Source: CAD feature listing. Evaluate the final solid. Frame: model axes, mm. A direction names the side the tool comes from. Give positions to 0.01 mm unless a question says otherwise; leave off trailing zeros. Write each loop counter-clockwise with the first axis right and the second up, starting at its lowest first coordinate (ties: lowest second). Pieces come first, ordered by that corner, then holes.
```python
from build123d import *

# Parameters (mm, degrees)
SKETCH2_R           = 1.5875
BOSS_EXTRUDE1_DEPTH = 1.6
SKETCH3_W           = 15.875
SKETCH3_H           = 16.4592
BOSS_EXTRUDE2_DEPTH = 12.5


with BuildPart() as part:
    # Sketch2 → Boss-Extrude1 (new body)
    with BuildSketch(Plane.XY):
        with BuildLine():
            Line((0, 4.1529), (14.986, 4.1529))
            Line((14.986, 4.1529), (14.986, 12.7762))
            Line((14.986, 12.7762), (33.3756, 12.7762))
            Line((33.3756, 12.7762), (33.3756, 4.445))
            Line((33.3756, 4.445), (41.3766, 4.445))
            Line((41.3766, 4.445), (41.3766, 11.0109))
            ThreePointArc((41.3766, 11.0109), (43.2181, 12.8524), (45.0596, 11.0109))
            Line((45.0596, 11.0109), (45.0596, 0))
            Line((45.0596, 0), (56.2864, 0))
            Line((56.2864, 0), (56.2864, 7.5819))
            ThreePointArc((56.2864, 7.5819), (57.1881, 8.4836), (58.0898, 7.5819))
            Line((58.0898, 7.5819), (58.0898, 0))
            Line((58.0898, 0), (65.3034, 0))
            Line((65.3034, 0), (65.3034, 44.6024))
            Line((65.3034, 44.6024), (0, 44.6024))
            Line((0, 44.6024), (0, 4.1529))
        make_face()
        with Locations((5.5245, 37.5285)):
            Circle(SKETCH2_R, mode=Mode.SUBTRACT)
        with Locations((5.55, 7.9883)):
            Circle(SKETCH2_R, mode=Mode.SUBTRACT)
    extrude(amount=BOSS_EXTRUDE1_DEPTH)

    # Sketch3 → Boss-Extrude2 (add)
    with BuildSketch(Plane.XY.offset(1.6)):
        with Locations((6.2103, 23.0124)):
            Rectangle(SKETCH3_W, SKETCH3_H)
    extrude(amount=BOSS_EXTRUDE2_DEPTH)


solid = part.part
```
1. Cut plane D-D, the plane x = 37. Return the cut outline in (y, z) (3 decimals).
2. Line query: L1, parallel to Y at x = 5.55, z = 0.5; L2, parallel to Z at x = 25, y = 37; L3, parallel to Y at x = 7, z = 3.75. Output: solid intervals per line, ascending.
3. Cut plane B-B, the plane x = 8. Return the cut outline in (y, z), then the cut area to 3 significant figures.
4. Mould query, pull axis X, two halves, no side actions, for faces 6 (the flat face through (39, 28, 1.6)), 7 (the cylindrical face through (43.178, 12.852, 0.789)), 8 (the flat face through (14.148, 23, 8)). Classes: +X half, -X half, draft (parallel to the pull), parting line (faces both ways), or undercut.
5. Contact query for flat-ended pins moving along their axis: P1, Ø0.5, axis at x = 4, z = 0.5, coming from the -Y side; P2, Ø0.8, axis at y = 8, z = 0.5, coming from the -X side; P3, Ø12, axis at x = 25, y = 17.5, coming from the +Z side. Output: stop coordinate, or through.
6. Access query for faces 1 (the flat face through (0, 25, 1)), 2 (the flat face through (56.286, 4, 1)), 3 (the flat face through (7, 4.153, 1)), 4 (the flat face through (6, 31.242, 8)), 5 (the flat face through (6, 14.783, 8)). Directions: +Z, -Z, +X, -X, +Y, -Y. A direction counts if a zero-diameter tool reaches every point of the face in a straight line with its end or side. Return the directions, or none.
7. Cut plane C-C, the plane z = 7. Return the cut outline in (x, y), then the cut area to 3 significant figures.
8. Cut plane A-A, the plane y = 30. Return the cut outline in (x, z).
Response values:
1. outline: (4.445, 0) - (44.602, 0) - (44.602, 1.6) - (4.445, 1.6) - close
2. L1: y = 4.15 to 6.4, 9.58 to 35.94, 39.12 to 44.6
2. L2: z = 0 to 1.6
2. L3: y = 14.78 to 31.24
3. outline: (4.15, 0) - (44.6, 0) - (44.6, 1.6) - (31.24, 1.6) - (31.24, 14.1) - (14.78, 14.1) - (14.78, 1.6) - (4.15, 1.6) - close
3. area: 270 mm2
4. face 6: draft
4. face 7: undercut
4. face 8: +X half
5. P1: stops at y = 4.15
5. P2: stops at x = 0
5. P3: stops at z = 1.6
6. face 1: -Z, -X, +Y, -Y
6. face 2: +Z, -Z, -Y
6. face 3: +Z, -Z, -X, -Y
6. face 4: +Z, +X, -X, +Y
6. face 5: +Z, +X, -X, -Y
7. outline: (-1.73, 14.78) - (14.15, 14.78) - (14.15, 31.24) - (-1.73, 31.24) - close
7. area: 261 mm2
8. outline: (-1.73, 1.6) - (0, 1.6) - (0, 0) - (65.3, 0) - (65.3, 1.6) - (14.15, 1.6) - (14.15, 14.1) - (-1.73, 14.1) - close
